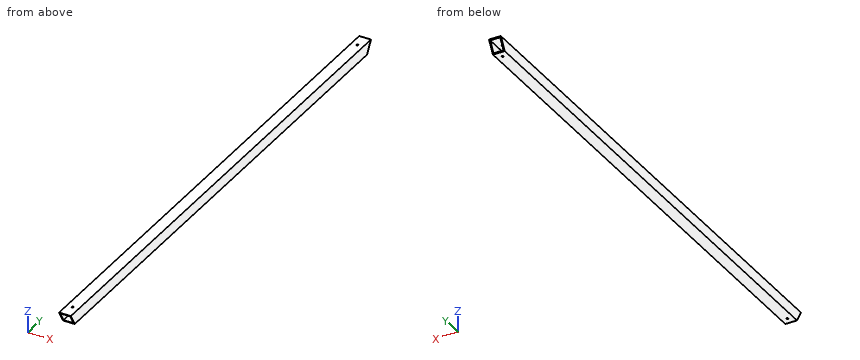
```python
from build123d import *

# Parameters (mm, degrees)
SKETCH1_W           = 44.45
SKETCH1_H           = 1980.184
BOSS_EXTRUDE1_DEPTH = 44.45
SKETCH2_W           = 38.1
SKETCH2_H           = 38.1
CUT_EXTRUDE1_DEPTH  = 1981.807518913
CUT_EXTRUDE2_DEPTH  = 993.085567612
SKETCH13_R          = 3.3734375
CUT_EXTRUDE7_DEPTH  = 992.338449567


with BuildPart() as part:
    # Sketch1 → Boss-Extrude1 (new body)
    with BuildSketch(Plane.XY):
        Rectangle(SKETCH1_W, SKETCH1_H)
    extrude(amount=BOSS_EXTRUDE1_DEPTH)

    # Sketch2 → Cut-Extrude1 (cut, through all)
    with BuildSketch(Plane(origin=(0, 990.092, 0), x_dir=(1, 0, 0), z_dir=(0, 1, 0))):
        with Locations((0, -22.225)):
            Rectangle(SKETCH2_W, SKETCH2_H)
    extrude(amount=-CUT_EXTRUDE1_DEPTH, mode=Mode.SUBTRACT)

    # Sketch3 → Cut-Extrude2 (cut, through all)
    with BuildSketch(Plane(origin=(22.225, 0, 0), x_dir=(0, 0, -1), z_dir=(1, 0, 0))):
        Polygon((-44.45, 990.092), (0, 964.428780535), (0, 990.092), align=None)
        Polygon((-44.45, -990.092), (0, -964.428780535), (0, -990.092), align=None)
    extrude(amount=-CUT_EXTRUDE2_DEPTH, mode=Mode.SUBTRACT)

    # Sketch13 → Cut-Extrude7 (cut, through all)
    with BuildSketch(Plane.XY.offset(44.45)):
        with Locations((0, 939.038)):
            Circle(SKETCH13_R)
        with Locations((0, -939.038)):
            Circle(SKETCH13_R)
    extrude(amount=-CUT_EXTRUDE7_DEPTH, mode=Mode.SUBTRACT)


solid = part.part
```
The model under review builds one solid part; all positions refer to its coordinate system, in mm. Round coordinates to 2 decimals unless told otherwise and drop trailing zeros. Write each loop counter-clockwise with the first axis right and the second up, starting at its lowest first coordinate (ties: lowest second). Pieces come first, ordered by that corner, then holes. Notation, with made-up numbers: (46, 74) - (62, 74) arc R15 cw to (62, 96) - close; hole circle Ø10 at (9, -6.5). An arc over 180 degrees is marked (long way). One line per question, with ' | ' between items.
Item 1: Add section B-B, the plane y = -731.5. Give the boundary of the cut face in (x, z) (3 decimals).
Resolved:
outline: (-22.225, 0) - (22.225, 0) - (22.225, 44.45) - (-22.225, 44.45) - close; hole (-19.05, 3.175) - (19.05, 3.175) - (19.05, 41.275) - (-19.05, 41.275) - close
Item 2: Add section C-C, the plane z = 34.5. Give the boundary of the cut face in (x, y) (3 decimals), then the cut area to 3 significant figures.
Resolved:
outline: (-22.225, -984.347) - (-19.05, -984.347) - (-19.05, 984.347) - (-22.225, 984.347) - close; (19.05, -984.347) - (22.225, -984.347) - (22.225, 984.347) - (19.05, 984.347) - close | area: 12,500 mm2
Item 3: Add section A-A, the plane x = 11.5. Give the boundary of the cut face in (y, z) (3 decimals).
Resolved:
outline: (-990.092, 44.45) - (-988.259, 41.275) - (988.259, 41.275) - (990.092, 44.45) - close; (-966.262, 3.175) - (-964.429, 0) - (964.429, 0) - (966.262, 3.175) - close
Item 4: To check wall thickness, follow probe 1 along Z at (x, y) = (-17.5, -70) (3 decimals); probe 2 along X at (y, z) = (77.5, 18) (3 decimals). State the ranges of each line that lie inside material, in increasing order.
Resolved:
probe 1: z = 0 to 3.175, 41.275 to 44.45 | probe 2: x = -22.225 to -19.05, 19.05 to 22.225
